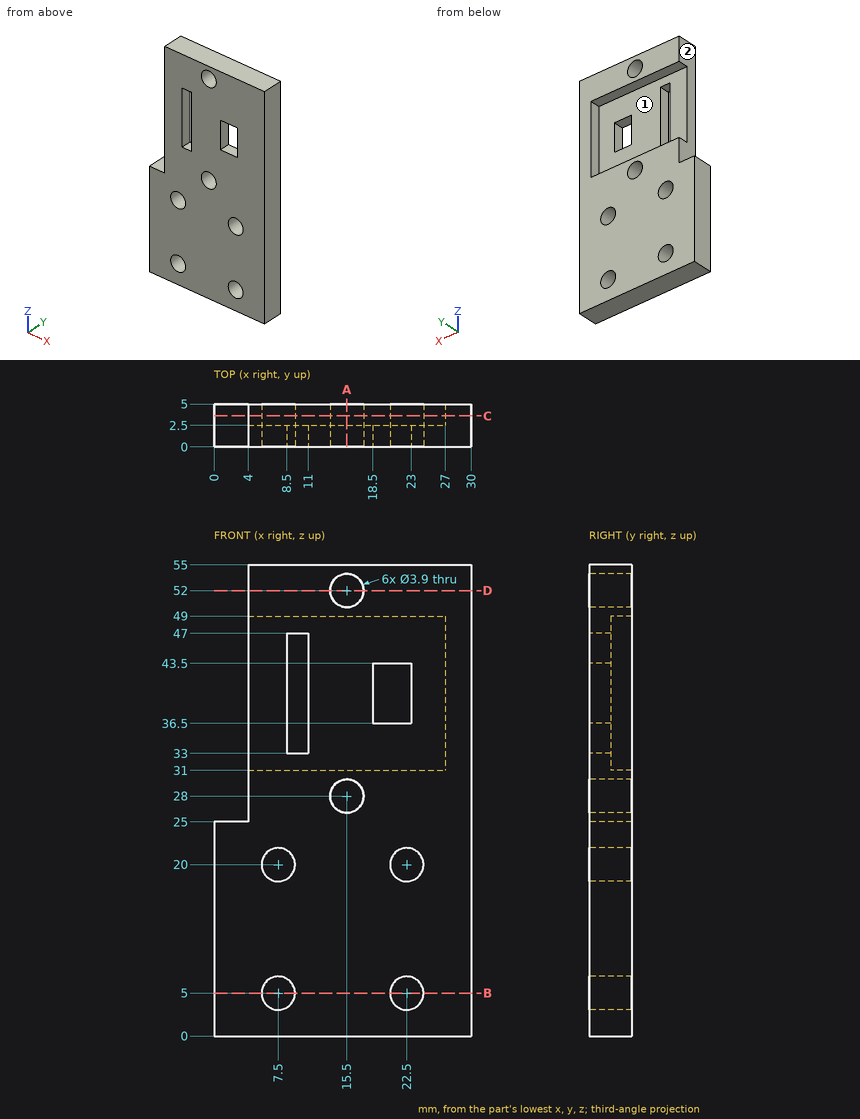
Design review of the part shown in the three views and the two pictorial views. Dimensions are in mm from the part's minimum x, y and z. Coordinates: 2 decimals unless noted, no trailing zeros. Loops run counter-clockwise (first coordinate to the right, second up) from the corner with the lowest first, then second, coordinate; pieces in that order, holes last.
Q1. We need section A-A on x = 15.5. State the section outline as (y, z) points, and give its area (3 significant figures).
Reported:
outline: (0, 0) - (5, 0) - (5, 26.05) - (0, 26.05) - close; (0, 29.95) - (5, 29.95) - (5, 31) - (2.5, 31) - (2.5, 49) - (5, 49) - (5, 50.05) - (0, 50.05) - close; (0, 53.95) - (5, 53.95) - (5, 55) - (0, 55) - close
area: 191 mm2
Q2. We need section C-C on y = 3.6. State the section outline as (x, z) points, and give its area (3 significant figures).
Reported:
outline: (0, 0) - (30, 0) - (30, 55) - (4, 55) - (4, 49) - (27, 49) - (27, 31) - (4, 31) - (4, 25) - (0, 25) - close; hole circle Ø3.9 at (7.5, 5); hole circle Ø3.9 at (7.5, 20); hole circle Ø3.9 at (15.5, 28); hole circle Ø3.9 at (15.5, 52); hole circle Ø3.9 at (22.5, 5); hole circle Ø3.9 at (22.5, 20)
area: 1,040 mm2
Q3. We need section D-D on z = 52. State the section outline as (x, y) points, and give its area (4 significant figures).
Reported:
outline: (4, 0) - (13.55, 0) - (13.55, 5) - (4, 5) - close; (17.45, 0) - (30, 0) - (30, 5) - (17.45, 5) - close
area: 110.5 mm2
Q4. To check wall thickness, follow line 1 (Z direction, x = 7.5, y = 2.8); line 2 (X direction, y = 3.65, z = 5); line 3 (Z direction, x = 15.5, y = 2.4). State the ranges of each line that lie inside material, in increasing order.
Reported:
line 1: z = 0 to 3.05, 6.95 to 18.05, 21.95 to 31, 49 to 55
line 2: x = 0 to 5.55, 9.45 to 20.55, 24.45 to 30
line 3: z = 0 to 26.05, 29.95 to 50.05, 53.95 to 55
Q5. For pin 1 (1.2 mm diameter, centred on x = 1.5, y = 1.5, fed in from +Z); pin 2 (3 mm diameter, centred on y = 4.5, z = 42, fed in from -X); pin 3 (3 mm diameter, centred on y = 1.5, z = 38, fed in from -X), all flat-tipped, find the tip position at first contact; note any pin that passes through.
Reported:
pin 1: stops at z = 25
pin 2: stops at x = 27
pin 3: stops at x = 4
Q6. We need section B-B on z = 5. State the section outline as (x, y) points.
Reported:
outline: (0, 0) - (5.55, 0) - (5.55, 5) - (0, 5) - close; (9.45, 0) - (20.55, 0) - (20.55, 5) - (9.45, 5) - close; (24.45, 0) - (30, 0) - (30, 5) - (24.45, 5) - close
Q7. The part is to be moulded in two halves that separate along Z. For the marked faces 1 and 2, say which applies: +Z half, -Z half, draft (parallel to the pull), parting line (faces both ways), or undercut.
Reported:
face 1: undercut
face 2: draft
